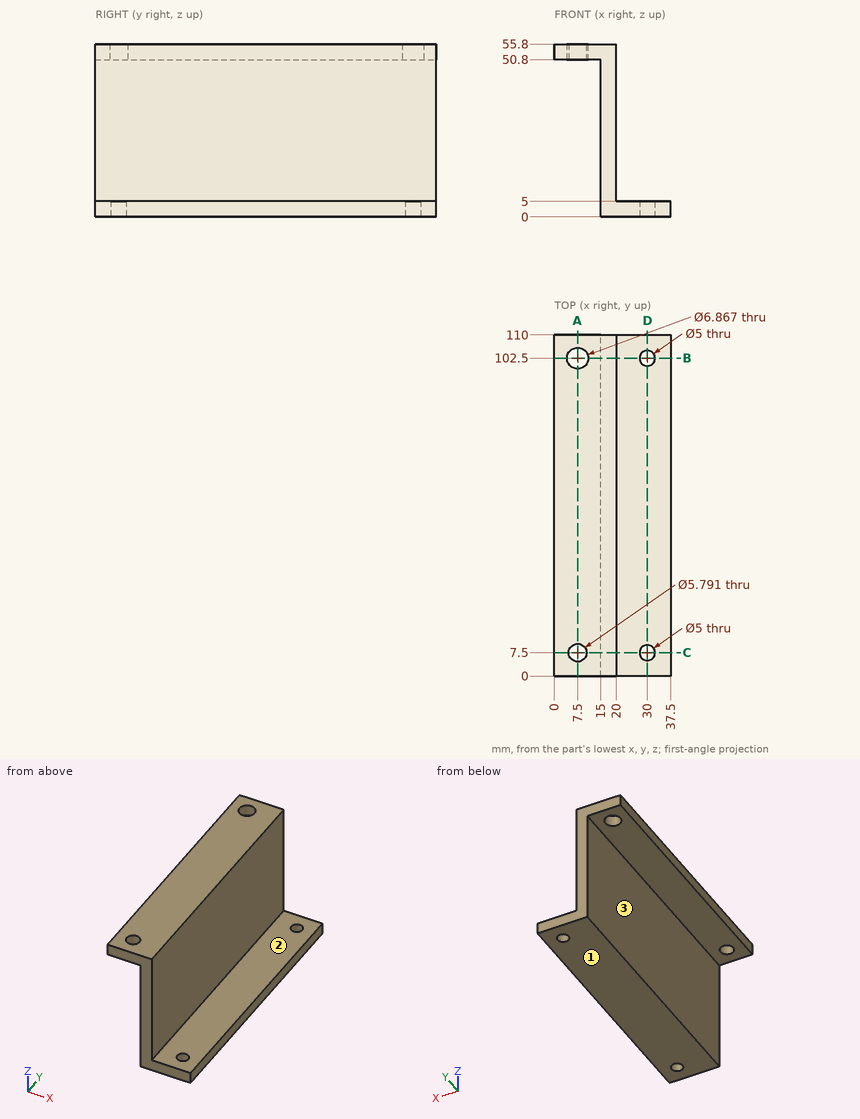
Geometry check sheet. Reference: drawing and pictorial views, mm from the part's lowest x, y, z. A direction names the side the tool comes from. Round coordinates to 2 decimals unless told otherwise and drop trailing zeros. Loops run counter-clockwise (first coordinate to the right, second up) from the corner with the lowest first, then second, coordinate; pieces in that order, holes last. Notation, with made-up numbers: (12, -30.75) -> (71, -30.75) arc R18 cw to (71, -18.75) -> close; hole circle Ø8 at (31.25, -34.75). An arc over 180 degrees is marked (long way). Answer as a JSON object with one key per item and string values. Group by question number.
Item 1: Cross-section at B-B, the plane y = 102.5. Record the cut outline in (x, z), plus the area to 3 significant figures.
Item 2: Cross-section at C-C, the plane y = 7.5. Record the cut outline in (x, z) (1 decimal).
Item 3: Thickness scan on line 1 along Y through (x, z) = (30, 3.85); line 2 along Y through (x, z) = (7.5, 54) (1 decimal); line 3 along X through (y, z) = (7.5, 54.45) (1 decimal). Record the ranges inside material, lowest first.
Item 4: Cross-section at A-A, the plane x = 7.5. Record the cut outline in (y, z) (1 decimal), plus the area to 3 significant figures.
Item 5: Depth check by flat-ended pin: pin 1 Ø3 at (y, z) = (47, 8.5) entering from -X; pin 2 Ø7.5 at (x, y) = (7.5, 7.5) entering from -Z; pin 3 Ø6 at (x, y) = (30, 102.5) entering from +Z. Enter the tip coordinate at first touch or a pass-through.
Item 6: Set-up check for the marked faces 1, 2 and 3: record each of +Z, -Z, +X, -X, +Y, -Y from which the full face is reachable in a straight line by a thin tool's end or side.
Item 7: Cross-section at D-D, the plane x = 30. Record the cut outline in (y, z).
Determined:
{
 "1": {"outline": "(0, 50.8) -> (4.07, 50.8) -> (4.07, 55.8) -> (0, 55.8) -> close; (10.93, 50.8) -> (15, 50.8) -> (15, 0) -> (27.5, 0) -> (27.5, 5) -> (20, 5) -> (20, 55.8) -> (10.93, 55.8) -> close; (32.5, 0) -> (37.5, 0) -> (37.5, 5) -> (32.5, 5) -> close", "area": "382 mm²"},
 "2": {"outline": "(0, 50.8) -> (4.6, 50.8) -> (4.6, 55.8) -> (0, 55.8) -> close; (10.4, 50.8) -> (15, 50.8) -> (15, 0) -> (27.5, 0) -> (27.5, 5) -> (20, 5) -> (20, 55.8) -> (10.4, 55.8) -> close; (32.5, 0) -> (37.5, 0) -> (37.5, 5) -> (32.5, 5) -> close"},
 "3": {"line 1": "y = 0 to 5, 10 to 100, 105 to 110", "line 2": "y = 0 to 4.6, 10.4 to 99.1, 105.9 to 110", "line 3": "x = 0 to 4.6, 10.4 to 20"},
 "4": {"outline": "(0, 50.8) -> (4.6, 50.8) -> (4.6, 55.8) -> (0, 55.8) -> close; (10.4, 50.8) -> (99.1, 50.8) -> (99.1, 55.8) -> (10.4, 55.8) -> close; (105.9, 50.8) -> (110, 50.8) -> (110, 55.8) -> (105.9, 55.8) -> close", "area": "487 mm²"},
 "5": {"pin 1": "stops at x = 15", "pin 2": "stops at z = 50.8", "pin 3": "stops at z = 5"},
 "6": {"face 1": "-Z, +X, -X, +Y, -Y", "face 2": "+Z, +X, +Y, -Y", "face 3": "-Z, -X, +Y, -Y"},
 "7": {"outline": "(0, 0) -> (5, 0) -> (5, 5) -> (0, 5) -> close; (10, 0) -> (100, 0) -> (100, 5) -> (10, 5) -> close; (105, 0) -> (110, 0) -> (110, 5) -> (105, 5) -> close"}
}
